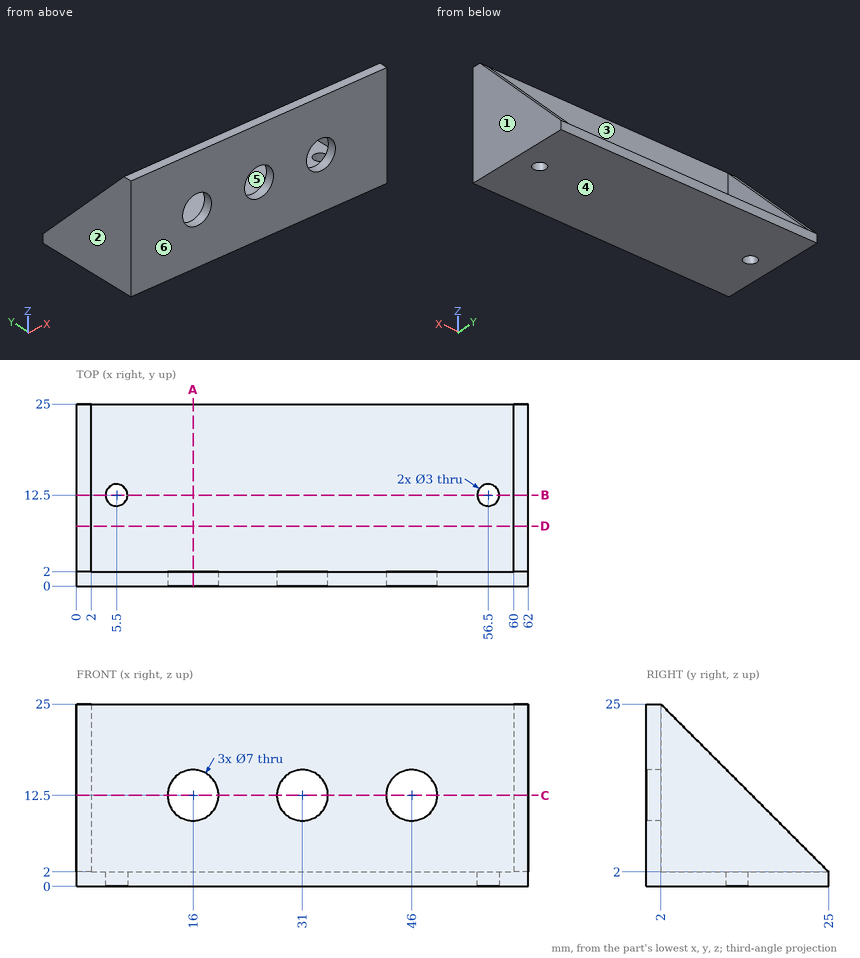
Answer from the drawing. Dimensions are ordinates in mm from the lowest x, y and z of the part. A direction names the side the tool comes from. Give positions to 0.01 mm unless a question says otherwise; leave off trailing zeros. Write each loop counter-clockwise with the first axis right and the second up, starting at its lowest first coordinate (ties: lowest second). Pieces come first, ordered by that corner, then holes. Notation, with made-up numbers: M 28,81 L 65,81 A21 ccw 65,116 Z; hole C 55,-18.5 d3. An arc over 180 degrees is marked long. Answer as CSV lines item,"result".
Q1. A tool of negligible diameter and unlimited length cuts with its end or side. For the marked faces 5 and 6, from which of +Z, -Z, +X, -X, +Y, -Y can it reach the whole face along a straight path? Write none if from no direction.
A:
face 5,"+Z, +Y"
face 6,"+Z, -Z, +X, -X, -Y"
Q2. A cutting plane is placed at D-D on y = 8.25. Write down the section's boundary in (x, z), plus the area to 3 significant figures.
A:
outline,"M 0,0 L 62,0 L 62,18.75 L 60,18.75 L 60,2 L 2,2 L 2,18.75 L 0,18.75 Z"
area,"191 mm²"
Q3. A cutting plane is placed at A-A on x = 16. Write down the section's boundary in (y, z).
A:
outline,"M 0,0 L 25,0 L 25,2 L 2,2 L 2,9 L 0,9 Z; M 0,16 L 2,16 L 2,25 L 0,25 Z"
Q4. A cutting plane is placed at B-B on y = 12.5. Write down the section's boundary in (x, z), plus the area to 3 significant figures.
A:
outline,"M 0,0 L 4,0 L 4,2 L 2,2 L 2,14.5 L 0,14.5 Z; M 7,0 L 55,0 L 55,2 L 7,2 Z; M 58,0 L 62,0 L 62,14.5 L 60,14.5 L 60,2 L 58,2 Z"
area,"162 mm²"
Q5. The mould has two halves that part along X. Classify the marked faces 1, 2, 3 and 4: +X half, -X half, draft (parallel to the pull), parting line (faces both ways), or undercut.
A:
face 1,"+X half"
face 2,"-X half"
face 3,"undercut"
face 4,"draft"
Q6. Given P1, Ø3, axis at x = 32.5, z = 18, coming from the +Y side; P2, Ø4, axis at x = 16, z = 12.5, coming from the +Y side, each flat-ended and moving along its own axis, determine where each tip first touches the part or whether it passes through.
A:
P1,"stops at y = 2"
P2,"passes through"
Q7. Find the intervals of material crossed by probe 1 along X at (y, z) = (4.75, 6.75); probe 2 along Y at (x, z) = (56.5, 1.4); probe 3 along X at (y, z) = (1.5, 12), in increasing order. Write a range as [from, to].
A:
probe 1,"x = [0, 2], [60, 62]"
probe 2,"y = [0, 11], [14, 25]"
probe 3,"x = [0, 12.54], [19.46, 27.54], [34.46, 42.54], [49.46, 62]"
Q8. A cutting plane is placed at C-C on z = 12.5. Write down the section's boundary in (x, y), plus the area to 3 significant figures.
A:
outline,"M 0,0 L 12.5,0 L 12.5,2 L 2,2 L 2,14.5 L 0,14.5 Z; M 19.5,0 L 27.5,0 L 27.5,2 L 19.5,2 Z; M 34.5,0 L 42.5,0 L 42.5,2 L 34.5,2 Z; M 49.5,0 L 62,0 L 62,14.5 L 60,14.5 L 60,2 L 49.5,2 Z"
area,"132 mm²"
